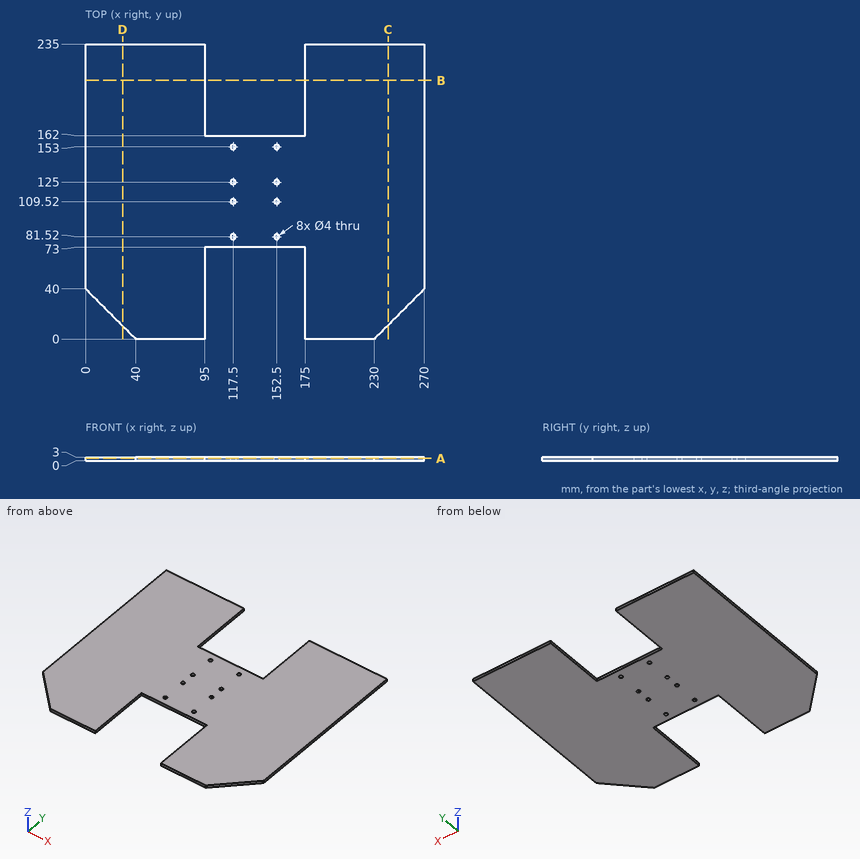
The drawing under review shows one solid part. Ordinate dimensions are in mm from its lowest x, y, z. Round coordinates to 2 decimals unless told otherwise and drop trailing zeros. Loops run counter-clockwise (first coordinate to the right, second up) from the corner with the lowest first, then second, coordinate; pieces in that order, holes last. Notation, with made-up numbers: M -26.75,-23.5 L 9.25,-23.5 A22 cw 9.25,-2.5 Z; hole C 71.5,20.25 d6. An arc over 180 degrees is marked long. Answer as CSV lines item,"result". Start each with the question number.
Item 1: Consider section A-A (z = 2). State how many separate pieces and enclosed holes the cut face has, then the cut area to 3 significant figures.
Item 2: Consider section D-D (x = 29.5). Write out the cut boundary in (y, z), then the cut area to 4 significant figures.
Item 3: Consider section B-B (y = 206). Write out the cut boundary in (x, z).
Item 4: Insertion check: P1, Ø0.9, axis at y = 21, z = 1.5, coming from the +X side; P2, Ø5, axis at x = 117.5, y = 81.52, coming from the +Z side; P3, Ø1.5, axis at x = 154, z = 1.5, coming from the +Y side; P4, Ø1.5, axis at x = 106.5, z = 1, coming from the -Y side. Each pin has a flat end and moves straight along its axis. Give the tip position at first contact, or say it passes through.
Item 5: Consider section C-C (x = 241). Write out the cut boundary in (y, z).
Item 6: Wall thickness on line 1 (Y direction, x = 117.5, z = 1.15); line 2 (X direction, y = 193.5, z = 1.75); line 3 (X direction, y = 16, z = 2.3): over which ranges is each line inside the solid? List them lowest first. Write a range as [from, to].
Answer:
1,separate pieces,"1"
1,enclosed holes,"8"
1,area,"50,100 mm^2"
2,outline,"M 10.5,0 L 235,0 L 235,3 L 10.5,3 Z"
2,area,"673.5 mm^2"
3,outline,"M 0,0 L 95,0 L 95,3 L 0,3 Z; M 175,0 L 270,0 L 270,3 L 175,3 Z"
4,P1,"stops at x = 251.45"
4,P2,"stops at z = 3"
4,P3,"stops at y = 162"
4,P4,"stops at y = 73"
5,outline,"M 11,0 L 235,0 L 235,3 L 11,3 Z"
6,line 1,"y = [73, 79.52], [83.52, 107.52], [111.52, 123], [127, 151], [155, 162]"
6,line 2,"x = [0, 95], [175, 270]"
6,line 3,"x = [24, 95], [175, 246]"
